Part model, mm, in its own coordinate system. Face numbers are marked on the shaded views. Give positions to 0.01 mm unless a question says otherwise; leave off trailing zeros. Order: outer loops, then holes, each group sorted by start corner. A loop starts at its lowest first (then second) coordinate and runs counter-clockwise, first axis right, second up.
from build123d import *

# Parameters (mm, degrees)
F1_DEPTH = 101.6
F2_T     = -2.54
F3_W     = 20.0663776208
F3_H     = 57.6037857682
F4_DEPTH = 50.8


with BuildPart() as f1:
    # F0 (on Top) → F1 (new body)
    with BuildSketch(Plane.XY):
        Polygon((32.0586711168, 25.0460729003), (-94.7746559978, 25.0460729003), (-90.6164767412, -44.7059123562), (32.2867780924, -44.3016439676), align=None)
    extrude(amount=F1_DEPTH)

    # F2
    f2_openings = [f1.faces().sort_by_distance(p)[0] for p in [
        (-31.357992, 25.046073, 50.8),
    ]]
    offset(amount=F2_T, openings=f2_openings)

    # F3 (on face) → F4 (cut)
    with BuildSketch(Plane(origin=(-92.951234691, -5.5411741264, 0), x_dir=(0.0595081302, -0.9982278209, 0), z_dir=(-0.9982278209, -0.0595081302, 0))):
        with Locations((-5.7368292903, 51.2475920841)):
            Rectangle(F3_W, F3_H)
    extrude(amount=-F4_DEPTH, mode=Mode.SUBTRACT)


solid = f1.part
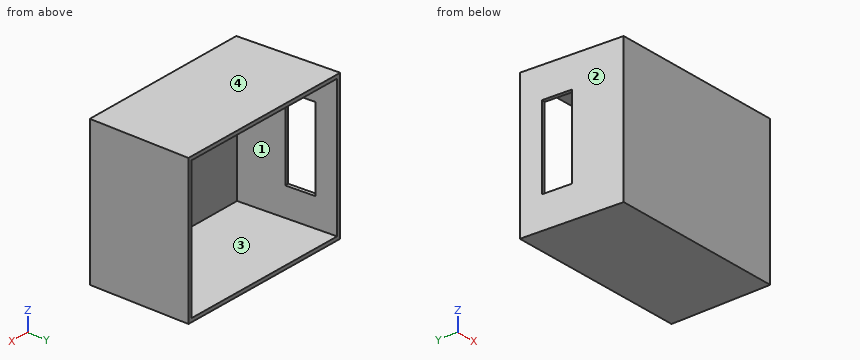
Item 1: Drill centre lines: probe 1 along Z at (x, y) = (-40.5, -37.5); probe 2 along X at (y, z) = (-17.5, 49); probe 3 along X at (y, z) = (-26, 55.5). Where is each one in solid material? Low to high.
Item 2: Drop flat-ended pins along their axis: P1, Ø6, axis at x = -55.5, z = 24.5, coming from the -Y side; P2, Ø3, axis at x = -91.5, y = 4, coming from the -Z side; P3, Ø3, axis at x = -73, z = 47, coming from the +Y side; P4, Ø10, axis at y = -10, z = 21.5, coming from the -X side. Give the stop position or say it passes through.
Item 3: Pull direction Z, two halves, no side cores. Call the marked faces 1, 2, 3 and 4: released by +Z, released by -Z, zero draft, split by the parting line, or undercut.
Item 4: Band-saw the part on A-A on z = 54. List the corners of the cut face in (x, y), plus the area to 3 significant figures.
Item 5: Band-saw the part on B-B on z = 94. List the corners of the cut face in (x, y), plus the area to 3 significant figures.
Item 6: Band-saw the part on D-D on y = -22. List the corners of the cut face in (x, z).
Item 7: Band-saw the part on C-C on x = -37.5. List the corners of the cut face in (y, z).
Working result:
1. probe 1: z = 0 to 2.54, 99.06 to 101.6
1. probe 2: x = -92.24 to -89.69, 29.66 to 32.2
1. probe 3: x = -91.73 to -89.19, 29.69 to 32.23
2. P1: stops at y = -44.6
2. P2: stops at z = 0
2. P3: stops at y = -42.1
2. P4: stops at x = -92.98
3. face 1: undercut
3. face 2: zero draft
3. face 3: undercut
3. face 4: released by +Z
4. outline: (-94.77, 25.05) - (-93.89, 10.2) - (-91.35, 10.35) - (-92.23, 25.05) - close; (-92.7, -9.83) - (-90.62, -44.71) - (32.29, -44.3) - (32.06, 25.05) - (29.52, 25.05) - (29.74, -41.77) - (-88.22, -42.16) - (-90.16, -9.68) - close
4. area: 602 mm2
5. outline: (-94.77, 25.05) - (-90.62, -44.71) - (32.29, -44.3) - (32.06, 25.05) - (29.52, 25.05) - (29.74, -41.77) - (-88.22, -42.16) - (-92.23, 25.05) - close
5. area: 653 mm2
6. outline: (-91.97, 0) - (32.21, 0) - (32.21, 101.6) - (-91.97, 101.6) - close; hole (-89.43, 2.54) - (29.67, 2.54) - (29.67, 99.06) - (-89.43, 99.06) - close
7. outline: (-44.53, 0) - (25.05, 0) - (25.05, 2.54) - (-41.99, 2.54) - (-41.99, 99.06) - (25.05, 99.06) - (25.05, 101.6) - (-44.53, 101.6) - close
